from build123d import *

# Parameters (mm, degrees)
SKETCH_1_R               = 78
SKETCH_1_R_2             = 63
EXTRUDE_1_DEPTH          = 4
SKETCH_2_R               = 2.05
CUT_EXTRUDE_1_DEPTH      = 4
PATTERN_CIRCULAR_1_COUNT = 10


with BuildPart() as part:
    # 草图1 → 凸台-拉伸1 (new body)
    with BuildSketch(Plane(origin=(0, 0, 0), x_dir=(1, 0, 0), z_dir=(0, 1, 0))):
        with Locations(Location((0, 0, 0), (0, 0, 270))):
            Circle(SKETCH_1_R)
        with Locations(Location((0, 0, 0), (0, 0, 270))):
            Circle(SKETCH_1_R_2, mode=Mode.SUBTRACT)
    extrude(amount=EXTRUDE_1_DEPTH)

    # 草图2 → 切除-拉伸1 (cut)
    with BuildSketch(Plane(origin=(0, 4, 0), x_dir=(1, 0, 0), z_dir=(0, 1, 0))):
        with Locations(Location((-72.1, 0, 0), (0, 0, 270))):
            Circle(SKETCH_2_R)
    cut_extrude_1 = extrude(amount=-CUT_EXTRUDE_1_DEPTH, mode=Mode.SUBTRACT)

    # 阵列(圆周)1: 切除-拉伸1 ×10 about axis
    pattern_circular_1_axis = Axis((0, 0, 0), (0, 1, 0))
    for i in range(1, PATTERN_CIRCULAR_1_COUNT):
        add(cut_extrude_1.rotate(pattern_circular_1_axis, i * 360 / PATTERN_CIRCULAR_1_COUNT), mode=Mode.SUBTRACT)


solid = part.part
Input: part model. Units: mm. Frame: model coordinates. Give positions to 0.01 mm unless a question says otherwise; leave off trailing zeros. Loops run counter-clockwise (first coordinate to the right, second up) from the corner with the lowest first, then second, coordinate; pieces in that order, holes last. Notation, with made-up numbers: (72.25, 45) - (97.25, 45) arc R13 cw to (97.25, 65) - close; hole circle Ø3 at (27.25, 78). An arc over 180 degrees is marked (long way). Use CSV: the item, a comma, the result in double quotes. Start each with the question number.
Item 1: Section D-D on y = 1.1. State how many separate pieces and enclosed holes the cut face has, then the cut area to 3 significant figures.
Item 2: Section B-B on x = 0. Return loops of the section in (y, z), then the cut area to 3 significant figures.
Item 3: Section A-A on z = 0. Return loops of the section in (x, y).
Item 4: Line query: line 1 (Z direction, x = 22, y = 3.15); line 2 (Z direction, x = -21, y = 2.4); line 3 (X direction, y = 2.75, z = 0). Output: solid intervals per line, ascending.
Item 5: Section C-C on z = 19.5. Return loops of the section in (x, y), then the cut area to 3 significant figures.
Item 6: Mould query, pull axis X, two halves, no side actions, for faces 1 (the flat face through (-63, 0, -6)), 2 (the cylindrical face through (77.336, 1.972, -10.154)), 3 (the cylindrical face through (-56.84, 2.03, 40.97)). Classes: pulls with the +X half, pulls with the -X half, needs draft (parallel to the pull), parting line crosses it, or undercut.
Item 7: Contact query for flat-ended pins moving along their axis: P1, Ø5.5, axis at x = 22.28, z = -68.57, coming from the -Y side; P2, Ø2, axis at y = 3.5, z = 0, coming from the +X side; P3, Ø3.5, axis at x = -58.33, z = -42.38, coming from the -Y side; P4, Ø1.5, axis at x = 57.5, y = 3, coming from the +Z side. Output: stop coordinate, or through.
Ans:
1,separate pieces,"1"
1,enclosed holes,"11"
1,area,"6,510 mm2"
2,outline,"(0, -78) - (4, -78) - (4, -63) - (0, -63) - close; (0, 63) - (4, 63) - (4, 78) - (0, 78) - close"
2,area,"120 mm2"
3,outline,"(-78, 0) - (-74.15, 0) - (-74.15, 4) - (-78, 4) - close; (-70.05, 0) - (-63, 0) - (-63, 4) - (-70.05, 4) - close; (63, 0) - (70.05, 0) - (70.05, 4) - (63, 4) - close; (74.15, 0) - (78, 0) - (78, 4) - (74.15, 4) - close"
4,line 1,"z = -74.83 to -70.6, -66.54 to -59.03, 59.03 to 66.54, 70.6 to 74.83"
4,line 2,"z = -75.12 to -70.17, -66.97 to -59.4, 59.4 to 66.97, 70.17 to 75.12"
4,line 3,"x = -78 to -74.15, -70.05 to -63, 63 to 70.05, 74.15 to 78"
5,outline,"(-75.52, 0) - (-59.91, 0) - (-59.91, 4) - (-75.52, 4) - close; (59.91, 0) - (75.52, 0) - (75.52, 4) - (59.91, 4) - close"
5,area,"125 mm2"
6,face 1,"needs draft"
6,face 2,"parting line crosses it"
6,face 3,"undercut"
7,P1,"stops at y = 0"
7,P2,"stops at x = 78"
7,P3,"passes through"
7,P4,"stops at z = 53.51"
